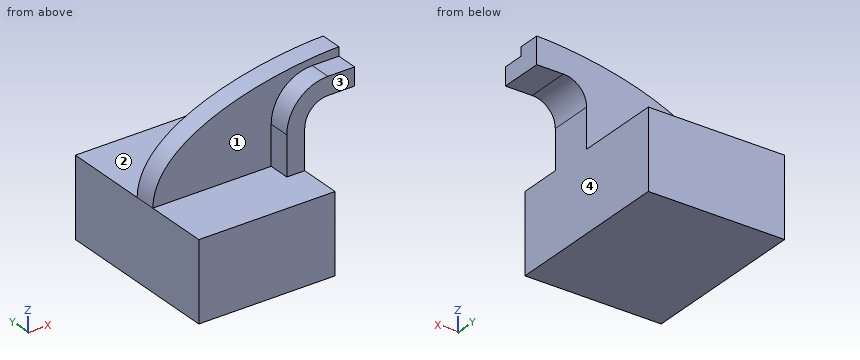
from build123d import *

# Parameters (mm, degrees)
F1_DEPTH = 50
F2_DEPTH = 25.4
F3_DEPTH = 12.7


with BuildPart() as f1:
    # F0 (on Front) → F1 (new body, symmetric)
    with BuildSketch(Plane.XZ):
        Polygon((39.676692, -22.906134), (39.676692, 22.906134), (29.262691, 22.906134), (-39.676692, 22.906134), (-39.676692, -22.906134), align=None)
    extrude(amount=F1_DEPTH, both=True)

    # F0 (on Front) → F2 (join)
    with BuildSketch(Plane.XZ):
        with BuildLine():
            Line((29.262691, 22.906134), (39.676692, 22.906134))
            Line((39.676692, 22.906134), (39.676692, 45.812268))
            ThreePointArc((39.676692, 45.812268), (43.628779, 55.35345), (53.169962, 59.305537))
            Line((53.169962, 59.305537), (68.718389, 59.305537))
            Line((68.718389, 59.305537), (68.718389, 69.719538))
            Line((68.718389, 69.719538), (53.169962, 69.719538))
            ThreePointArc((53.169962, 69.719538), (36.264969, 62.717261), (29.262691, 45.812268))
            Line((29.262691, 45.812268), (29.262691, 22.906134))
        make_face()
    extrude(amount=F2_DEPTH)

    # F0 (on Front) → F3 (join)
    with BuildSketch(Plane.XZ):
        with BuildLine():
            Line((-39.676692, 22.906134), (29.262691, 22.906134))
            Line((29.262691, 22.906134), (29.262691, 45.812268))
            ThreePointArc((29.262691, 45.812268), (36.264969, 62.717261), (53.169962, 69.719538))
            Line((53.169962, 69.719538), (68.718389, 69.719538))
            Line((68.718389, 69.719538), (68.718389, 74.853972))
            add(Edge.make_bspline(
                [(-39.676692, 22.906134), (-38.920954, 61.494272), (33.526827, 74.314252), (68.718389, 74.853972)],
                knots=[0, 0, 0, 0, 120.200131, 120.200131, 120.200131, 120.200131], degree=3))
        make_face()
    extrude(amount=F3_DEPTH)


solid = f1.part
Geometry: final body of the model. Coordinates: model frame, mm. Face numbers are marked on the shaded views. A direction names the side the tool comes from. Give positions to 0.01 mm unless a question says otherwise; leave off trailing zeros. Loops run counter-clockwise (first coordinate to the right, second up) from the corner with the lowest first, then second, coordinate; pieces in that order, holes last. Notation, with made-up numbers: (26, -29.75) - (42, -29.75) arc R19 cw to (42, -16.75) - close; hole circle Ø7 at (21, 53.25). An arc over 180 degrees is marked (long way). Answer as CSV lines item,"result". Start each with the question number.
1. Ray query, L1, parallel to X at y = 32.5, z = -12; L2, parallel to Z at x = 5.5, y = -39.5; L3, parallel to Y at x = -24, z = 25.5. Return the intervals inside material, ascending.
2. Section B-B, the plane z = 7.5. Return loops of the section in (x, y).
3. Pin query (flat end, axial travel): P1, Ø1, axis at x = -10.5, z = 49.5, coming from the -Y side; P2, Ø10, axis at x = -18, y = 0, coming from the +Z side; P3, Ø10, axis at y = -17, z = 37, coming from the -X side. Return the tip coordinate at first contact, or that it passes through.
4. Section A-A, the plane y = 41.5. Return loops of the section in (x, z).
5. Reachability of the marked faces 1, 2, 3 and 4 from +Z, -Z, +X, -X, +Y, -Y: full face, straight path, thin tool, end or side. Return the list, or none.
Answers:
1,L1,"x = -39.68 to 39.68"
1,L2,"z = -22.91 to 22.91"
1,L3,"y = -12.7 to 0"
2,outline,"(-39.68, -50) - (39.68, -50) - (39.68, 50) - (-39.68, 50) - close"
3,P1,"stops at y = -12.7"
3,P2,"stops at z = 56.86"
3,P3,"stops at x = -37.09"
4,outline,"(-39.68, -22.91) - (39.68, -22.91) - (39.68, 22.91) - (-39.68, 22.91) - close"
5,face 1,"+Z, -X, -Y"
5,face 2,"+Z, +X, -X, +Y"
5,face 3,"+Z, +X, -X, -Y"
5,face 4,"-Z, +X, +Y, -Y"
